```python
from build123d import *

# Parameters (mm, degrees)
SKETCH3_W               = 30
SKETCH3_H               = 22
BOSS_EXTRUDE1_DEPTH     = 1.5
SKETCH4_W               = 0.6
SKETCH4_H               = 22
BOSS_EXTRUDE2_DEPTH     = 10
CUT_EXTRUDE1_DEPTH      = 1
CUT_EXTRUDE1_DEPTH_BACK = 31
SKETCH6_W               = 30
SKETCH6_H               = 11.5
BOSS_EXTRUDE3_DEPTH     = 1.6
SKETCH7_W               = 13.6
SKETCH7_H               = 14.5
CUT_EXTRUDE2_DEPTH      = 1.6
FILLET1_R               = 2
SKETCH8_R               = 1.5
SKETCH8_R_2             = 1
CUT_EXTRUDE3_DEPTH      = 1.6


with BuildPart() as part:
    # Sketch3 → Boss-Extrude1 (new body)
    with BuildSketch(Plane.XY):
        Rectangle(SKETCH3_W, SKETCH3_H)
    extrude(amount=BOSS_EXTRUDE1_DEPTH)

    # Sketch4 → Boss-Extrude2 (add)
    with BuildSketch(Plane.XY.offset(1.5)):
        with Locations((-14.7, 0)):
            Rectangle(SKETCH4_W, SKETCH4_H)
    boss_extrude2 = extrude(amount=BOSS_EXTRUDE2_DEPTH)

    # Mirror5: Boss-Extrude2 across plane
    add(boss_extrude2.mirror(Plane(origin=(0, 0, 0), x_dir=(0, 0, 1), z_dir=(1, 0, 0))))

    # Sketch5 → Cut-Extrude1 (cut, two sides)
    with BuildSketch(Plane.ZY.offset(15)) as cut_extrude1_sk:
        Polygon((-16.404677134, 62.110913313), (5.5, 11), (11.5, -3), (33.404677134, -54.110913313), (135.626503761, -10.301559045), (85.817149492, 105.920267582), align=None)
    extrude(amount=CUT_EXTRUDE1_DEPTH, mode=Mode.SUBTRACT)
    extrude(cut_extrude1_sk.sketch, amount=-CUT_EXTRUDE1_DEPTH_BACK, mode=Mode.SUBTRACT)

    # Sketch6 → Boss-Extrude3 (add)
    with BuildSketch(Plane.XZ.offset(11)):
        with Locations((0, 5.75)):
            Rectangle(SKETCH6_W, SKETCH6_H)
    extrude(amount=BOSS_EXTRUDE3_DEPTH)

    # Sketch7 → Cut-Extrude2 (cut)
    with BuildSketch(Plane.XY.offset(1.5)):
        with Locations((0, 3.75)):
            Rectangle(SKETCH7_W, SKETCH7_H)
    extrude(amount=-CUT_EXTRUDE2_DEPTH, mode=Mode.SUBTRACT)

    # Fillet1
    fillet1_edges = [part.edges().sort_by_distance(p)[0] for p in [
        (-6.8, -3.5, 0.75),
        (6.8, -3.5, 0.75),
    ]]
    fillet(fillet1_edges, radius=FILLET1_R)

    # Sketch8 → Cut-Extrude3 (cut)
    with BuildSketch(Plane(origin=(0, -11, 0), x_dir=(1, 0, 0), z_dir=(0, 1, 0))):
        with Locations((0, -6.5)):
            Circle(SKETCH8_R)
        with Locations((-5, -6.5)):
            Circle(SKETCH8_R_2)
        with Locations((-10, -6.5)):
            Circle(SKETCH8_R)
        with Locations((5, -6.5)):
            Circle(SKETCH8_R_2)
        with Locations((10, -6.5)):
            Circle(SKETCH8_R)
    extrude(amount=-CUT_EXTRUDE3_DEPTH, mode=Mode.SUBTRACT)


solid = part.part
```
Verification items for the finished model (mm, model axes). A direction names the side the tool comes from. Round coordinates to 2 decimals unless told otherwise and drop trailing zeros. Write each loop counter-clockwise with the first axis right and the second up, starting at its lowest first coordinate (ties: lowest second). Pieces come first, ordered by that corner, then holes. Notation, with made-up numbers: (-35.5, 48) -> (14.5, 48) arc R14 ccw to (14.5, 60) -> close; hole circle Ø1 at (-20.5, -23.75). An arc over 180 degrees is marked (long way). Write each question's results on one line, items separated by ' | '. Start each with the question number.
1. Set-up check for faces 1 (the cylindrical face through (4.87, -11.79, 5.51)), 2 (the cylindrical face through (-6.23, -2.9, 0.74)), 3 (the flat face through (0, -11, 9)): record each of +Z, -Z, +X, -X, +Y, -Y from which the full face is reachable in a straight line by a thin tool's end or side.
2. Material ranges on probe 1 along X at (y, z) = (-11.85, 6.5); probe 2 along X at (y, z) = (-5.25, 8.75); probe 3 along Z at (x, y) = (0, -11.55), recorded low to high. Write a range as from..to.
3. Cross-section at B-B (z = 1). Enter the section's corners in (x, y).
4. Depth check by flat-ended pin: P1, Ø2, axis at x = 7, y = 6, coming from the -Z side; P2, Ø6.5, axis at x = -5.5, y = 1.5, coming from the +Z side; P3, Ø3, axis at x = -1.5, z = 8, coming from the +Y side; P4, Ø0.8, axis at x = -2, z = 1, coming from the +Y side. Enter the tip coordinate at first touch or a pass-through.
5. Cross-section at D-D (z = 6.5). Enter the section's corners in (x, y).
6. Cross-section at A-A (x = 0). Enter the section's corners in (y, z), then the cut area to 4 significant figures.
7. Cross-section at C-C (y = 4.75). Enter the section's corners in (x, z).
8. Draft check along Z on faces 4 (the cylindrical face through (8.8, -11.8, 7.4)), 5 (the flat face through (12, 11, 1)), 6 (the flat face through (0, -6, 0)). Enter one of: +Z half, -Z half, draft (parallel to the pull), parting line (faces both ways), or undercut.
Solutions:
1) face 1: +Y, -Y | face 2: +Z, -Z, +Y | face 3: +Z, +Y
2) probe 1: x = -15..-11.5, -8.5..-6, -4..-1.5, 1.5..4, 6..8.5, 11.5..15 | probe 2: x = -15..-14.4, 14.4..15 | probe 3: z = 0..5, 8..11.5
3) outline: (-15, -12.6) -> (15, -12.6) -> (15, 11) -> (6.8, 11) -> (6.8, -1.5) arc R2 cw to (4.8, -3.5) -> (-4.8, -3.5) arc R2 cw to (-6.8, -1.5) -> (-6.8, 11) -> (-15, 11) -> close
4) P1: stops at z = 0 | P2: stops at z = 1.5 | P3: stops at y = -11 | P4: stops at y = -3.5
5) outline: (-15, -12.6) -> (-11.5, -12.6) -> (-11.5, -11) -> (-14.4, -11) -> (-14.4, 8.67) -> (-15, 8.67) -> close; (-8.5, -12.6) -> (-6, -12.6) -> (-6, -11) -> (-8.5, -11) -> close; (-4, -12.6) -> (-1.5, -12.6) -> (-1.5, -11) -> (-4, -11) -> close; (1.5, -12.6) -> (4, -12.6) -> (4, -11) -> (1.5, -11) -> close; (6, -12.6) -> (8.5, -12.6) -> (8.5, -11) -> (6, -11) -> close; (11.5, -12.6) -> (15, -12.6) -> (15, 8.67) -> (14.4, 8.67) -> (14.4, -11) -> (11.5, -11) -> close
6) outline: (-12.6, 0) -> (-3.5, 0) -> (-3.5, 1.5) -> (-11, 1.5) -> (-11, 5) -> (-12.6, 5) -> close; (-12.6, 8) -> (-11, 8) -> (-11, 11.5) -> (-12.6, 11.5) -> close | area: 24.85 mm2
7) outline: (-15, 0) -> (-6.8, 0) -> (-6.8, 1.5) -> (-14.4, 1.5) -> (-14.4, 8.18) -> (-15, 8.18) -> close; (6.8, 0) -> (15, 0) -> (15, 8.18) -> (14.4, 8.18) -> (14.4, 1.5) -> (6.8, 1.5) -> close
8) face 4: undercut | face 5: draft | face 6: -Z half
